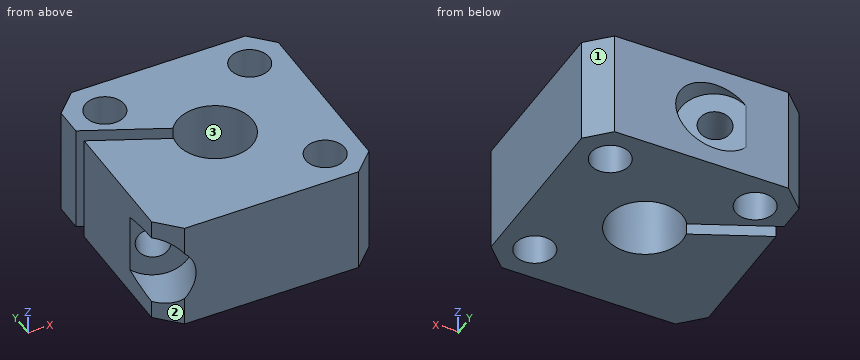
```python
from build123d import *

# Parameters (mm, degrees)
F0_W      = 30
F0_H      = 30
F0_R      = 2.7
F0_R_2    = 5.2
F1_DEPTH  = 15
F2_SIZE   = 3
F4_DEPTH  = 25
F5_R      = 2.2
F6_DEPTH  = 35
F8_R      = 5
F9_DEPTH  = 25
F11_R     = 5
F12_DEPTH = 25


with BuildPart() as f1:
    # F0 (on Top) → F1 (new body)
    with BuildSketch(Plane.XY):
        Rectangle(F0_W, F0_H)
        with Locations((10, -10)):
            Circle(F0_R, mode=Mode.SUBTRACT)
        with Locations((-10, 10)):
            Circle(F0_R, mode=Mode.SUBTRACT)
        Circle(F0_R_2, mode=Mode.SUBTRACT)
        with Locations((10, 10)):
            Circle(F0_R, mode=Mode.SUBTRACT)
    extrude(amount=F1_DEPTH)

    # F2
    f2_edges = [f1.edges().sort_by_distance(p)[0] for p in [
        (15, 15, 7.5),
        (15, -15, 7.5),
        (-15, -15, 7.5),
        (-15, 15, 7.5),
    ]]
    chamfer(f2_edges, length=F2_SIZE)

    # F3 (on face) → F4 (cut)
    with BuildSketch(Plane.XY.offset(15)):
        Polygon((-29.3442261462, 14.7868152936), (-29.7668444079, 13.8805075065), (-30.1894626697, 12.9741997195), (-3.0002290586, 0.2956518673), (-2.1549925351, 2.1082674413), align=None)
    extrude(amount=-F4_DEPTH, mode=Mode.SUBTRACT)

    # F5 (on face) → F6 (cut, symmetric)
    with BuildSketch(Plane(origin=(0.4226182617, 0.906307787, 0), x_dir=(0.906307787, -0.4226182617, 0), z_dir=(-0.4226182617, -0.906307787, 0))):
        with Locations((-8.1029403289, 7.5)):
            Circle(F5_R)
    extrude(amount=F6_DEPTH, both=True, mode=Mode.SUBTRACT)

    # F8 (on offset) → F9 (cut)
    with BuildSketch(Plane(origin=(4.6488008791, 9.9693856574, 0), x_dir=(0.906307787, -0.4226182617, 0), z_dir=(-0.4226182617, -0.906307787, 0))):
        with Locations((-8.1029403289, 7.5)):
            Circle(F8_R)
    extrude(amount=-F9_DEPTH, mode=Mode.SUBTRACT)

    # F11 (on offset) → F12 (cut)
    with BuildSketch(Plane(origin=(-5.0714191409, -10.8756934444, 0), x_dir=(0.906307787, -0.4226182617, 0), z_dir=(-0.4226182617, -0.906307787, 0))):
        with Locations((-8.1029403289, 7.5)):
            Circle(F11_R)
    extrude(amount=F12_DEPTH, mode=Mode.SUBTRACT)


solid = f1.part
```
Geometry: final body of the model. Coordinates: model frame, mm. Face numbers are marked on the shaded views. Round coordinates to 2 decimals unless told otherwise and drop trailing zeros. Loops run counter-clockwise (first coordinate to the right, second up) from the corner with the lowest first, then second, coordinate; pieces in that order, holes last. Notation, with made-up numbers: (61.5, 44) -> (89.5, 44) arc R16 cw to (89.5, 68) -> close; hole circle Ø2 at (48, 21.25). An arc over 180 degrees is marked (long way). Use one line per item in the form item = value.
Item 1: Cut plane D-D on y = 9.25. Give the number of separate pieces and of enclosed holes in the cut face, then the cut area to 3 significant figures.
Evaluation:
separate_pieces = 3
enclosed_holes = 1
area = 278 mm2
Item 2: Cut plane C-C on x = 4.5. Output: boundary loops of the cut face in (y, z), then the cut area to 3 significant figures.
Evaluation:
outline = (-15, 0) -> (-2.61, 0) -> (-2.61, 15) -> (-15, 15) -> close; (2.61, 0) -> (15, 0) -> (15, 15) -> (2.61, 15) -> close
area = 372 mm2
Item 3: Cut plane B-B on z = 8. Output: boundary loops of the cut face in (x, y).
Evaluation:
outline = (-15, -6.25) -> (-14.36, -6.55) -> (-9.71, 3.42) -> (-15, 5.89) -> close; (-15, 8.1) -> (-8.86, 5.24) -> (-4.64, 14.3) -> (-6.14, 15) -> (-12, 15) -> (-15, 12) -> close; (-10.47, -8.36) -> (-7.91, -9.55) -> (-10.45, -15) -> (12, -15) -> (15, -12) -> (15, 12) -> (12, 15) -> (3.54, 15) -> (1.81, 11.29) -> (-0.75, 12.49) -> (-4.98, 3.43) -> (-4.2, 3.06) arc R5.2 cw (long way) to (-5.05, 1.25) -> (-5.82, 1.61) -> close; hole circle Ø5.4 at (-10, 10); hole circle Ø5.4 at (10, -10); hole circle Ø5.4 at (10, 10)
Item 4: Contact query for a flat-ended pin moving along its axis: pin 1 Ø3 at (x, z) = (-2.5, 6.5) entering from +Y. Output: stop coordinate, or through.
Evaluation:
pin_1 = 13.86
Item 5: Material intervals for probe 1 along Y at (x, z) = (10, 11); probe 2 along X at (y, z) = (8.5, 14.25) (3 decimals); probe 3 along X at (y, z) = (-3.25, 8), sorted ascending.
Evaluation:
probe_1 = -15 to -12.7, -7.3 to 7.3, 12.7 to 15
probe_2 = -15 to -12.245, -7.755 to 7.755, 12.245 to 15
probe_3 = -15 to -12.82, -8.09 to -4.06, 4.06 to 15
Item 6: Draft query along Y for the marked faces 1, 2 and 3. Return one class per face: released by +Y, released by -Y, zero draft, split by the parting line, or undercut.
Evaluation:
face_1 = released by +Y
face_2 = released by -Y
face_3 = undercut
Item 7: Cut plane A-A on x = 10. Output: boundary loops of the cut face in (y, z).
Evaluation:
outline = (-15, 0) -> (-12.7, 0) -> (-12.7, 15) -> (-15, 15) -> close; (-7.3, 0) -> (7.3, 0) -> (7.3, 15) -> (-7.3, 15) -> close; (12.7, 0) -> (15, 0) -> (15, 15) -> (12.7, 15) -> close
